Input: dimensioned drawing with shaded views. Units: mm. Origin: part minimum x, y, z. Round coordinates to 2 decimals unless told otherwise and drop trailing zeros. Order: outer loops, then holes, each group sorted by start corner. A loop starts at its lowest first (then second) coordinate and runs counter-clockwise, first axis right, second up.
Item 1: Cut plane C-C on y = 2.95. Output: boundary loops of the cut face in (x, z), then the cut area to 3 significant figures.
Item 2: Cut plane B-B on x = 52.5. Output: boundary loops of the cut face in (y, z), then the cut area to 3 significant figures.
Item 3: First-contact query: pin 1 (6 mm diameter, centred on x = 12.5, z = 29.25, fed in from -Y). Flat tip, straight axial feed; report the tip coordinate or a pass-through.
Item 4: Cut plane A-A on z = 29.25. Output: boundary loops of the cut face in (x, y), then the cut area to 3 significant figures.
Item 5: Line query: L1, parallel to X at y = 3.05, z = 29.5; L2, parallel to X at y = 0.9, z = 31; L3, parallel to Z at x = 10.5, y = 2.4. Output: solid intervals per line, ascending.
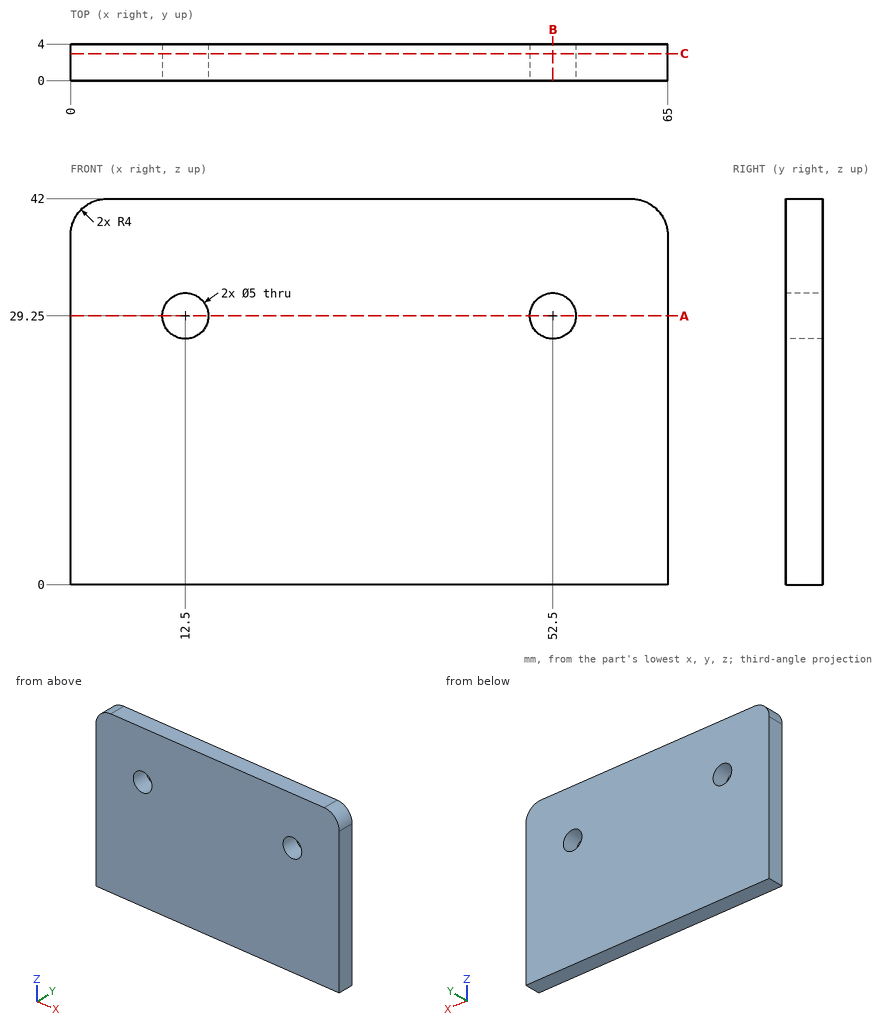
From the geometry:
1. outline: (0, 0) - (65, 0) - (65, 38) arc R4 ccw to (61, 42) - (4, 42) arc R4 ccw to (0, 38) - close; hole circle Ø5 at (12.5, 29.25); hole circle Ø5 at (52.5, 29.25)
1. area: 2,680 mm2
2. outline: (0, 0) - (4, 0) - (4, 26.75) - (0, 26.75) - close; (0, 31.75) - (4, 31.75) - (4, 42) - (0, 42) - close
2. area: 148 mm2
3. pin 1: stops at y = 0
4. outline: (0, 0) - (10, 0) - (10, 4) - (0, 4) - close; (15, 0) - (50, 0) - (50, 4) - (15, 4) - close; (55, 0) - (65, 0) - (65, 4) - (55, 4) - close
4. area: 220 mm2
5. L1: x = 0 to 10.01, 14.99 to 50.01, 54.99 to 65
5. L2: x = 0 to 10.71, 14.29 to 50.71, 54.29 to 65
5. L3: z = 0 to 27.75, 30.75 to 42
